The listing builds one solid part. Answer for the finished solid, in the listing's coordinates (mm). A direction names the side the tool comes from. Coordinates: 2 decimals unless noted, no trailing zeros. Loops run counter-clockwise (first coordinate to the right, second up) from the corner with the lowest first, then second, coordinate; pieces in that order, holes last. Notation, with made-up numbers: M -10,77 L 13,77 A34 cw 13,116 Z; hole C 57.5,11 d2. An arc over 180 degrees is marked long. Return JSON: item names as keys, results as strings. Group by question number.
1. Section A-A (x = -78) is taken. Write down the section's boundary in (y, z).
2. Section B-B (y = -24.5) is taken. Write down the section's boundary in (x, z), then the cut area to 3 significant figures.
3. Section D-D (y = 97.5) is taken. Write down the section's boundary in (x, z), then the cut area to 3 significant figures.
4. Which of the six approach directions +Z, -Z, +X, -X, +Y, -Y give full straight-line access (tool end or side, diameter ignored) to faces 5 (the face through (54.8, 38, 0.5)), 6 (the face through (-46, 32, 1))?
5. Straight lines are drawn through the part: L1, parallel to X at y = -25, z = 0.9; L2, parallel to X at y = -42.5, z = 0.3; L3, parallel to Y at x = -80.5, z = 0.65. For each, find the intervals that lie inside material, in ascending order. Write a range as from..to.
6. The mould has two halves that part along X. Classify faces 1 (the face through (-91, -49, 0.5)), 2 (the face through (104.27, -47.94, 0.49)), 3 (the face through (-46, 32, 0)), 4 (the face through (6.155, -50.41, 0.493)): pulls with the +X half, pulls with the -X half, needs draft (parallel to the pull), parting line crosses it, or undercut.
7. Section C-C (x = -172) is taken. Write down the section's boundary in (y, z).
```python
from build123d import *

# Parameters (mm, degrees)
ESQUISSE2_R             = 21.716757685
BOSS_EXTRU_1_DEPTH      = 1
ENL_V_MAT_EXTRU_2_DEPTH = 293.837814183
CONG_2_R                = 10
CONG_3_R                = 6
CONG_4_R                = 6
CONG_5_R                = 6


with BuildPart() as part:
    # Esquisse2 → Boss.-Extru.1 (new body)
    with BuildSketch(Plane.XY):
        with Locations((-43.22899501, 36.585487108)):
            Circle(ESQUISSE2_R)
        with BuildLine():
            ThreePointArc((-207.546192285, -7.001881243), (-132.259115873, 40.696309579), (-43.22899501, 36.585487108))
            ThreePointArc((-43.22899501, 36.585487108), (-84.183978752, -42.572270496), (-163.135361924, -83.923695834))
            ThreePointArc((-163.135361924, -83.923695834), (-190.453313653, -48.414512892), (-207.546192285, -7.001881243))
        make_face()
        with BuildLine():
            ThreePointArc((76.677371904, -83.923695834), (-2.274011269, -42.572270496), (-43.22899501, 36.585487108))
            ThreePointArc((-43.22899501, 36.585487108), (45.801125853, 40.696309579), (121.088202265, -7.001881243))
            ThreePointArc((121.088202265, -7.001881243), (103.995323633, -48.414512892), (76.677371904, -83.923695834))
        make_face()
        with BuildLine():
            Line((-43.22899501, 206.585487108), (-43.22899501, 58.302244794))
            ThreePointArc((-43.22899501, 58.302244794), (-34.753748483, 56.580180421), (-27.622617897, 51.687094896))
            ThreePointArc((-27.622617897, 51.687094896), (7.298277527, 122.217794206), (1.181835351, 200.682038403))
            ThreePointArc((1.181835351, 200.682038403), (-20.82825529, 205.103162324), (-43.22899501, 206.585487108))
        make_face()
        with BuildLine():
            ThreePointArc((-58.835372123, 51.687094896), (-51.704241537, 56.580180421), (-43.22899501, 58.302244794))
            Line((-43.22899501, 58.302244794), (-43.22899501, 206.585487108))
            ThreePointArc((-43.22899501, 206.585487108), (-65.62973473, 205.103162324), (-87.639825371, 200.682038403))
            ThreePointArc((-87.639825371, 200.682038403), (-93.756267547, 122.217794206), (-58.835372123, 51.687094896))
        make_face()
        with BuildLine():
            ThreePointArc((-48.504182436, 15.519164174), (-45.480177087, 25.955564863), (-43.22899501, 36.585487108))
            ThreePointArc((-43.22899501, 36.585487108), (-53.560368754, 39.950867364), (-64.110559549, 42.550202255))
            ThreePointArc((-64.110559549, 42.550202255), (-62.036258854, 25.727108266), (-48.504182436, 15.519164174))
        make_face()
        with BuildLine():
            ThreePointArc((-22.347430471, 42.550202255), (-32.897621267, 39.950867364), (-43.22899501, 36.585487108))
            ThreePointArc((-43.22899501, 36.585487108), (-40.977812933, 25.955564863), (-37.953807584, 15.519164174))
            ThreePointArc((-37.953807584, 15.519164174), (-26.109159563, 23.224020174), (-21.512237325, 36.585487108))
            ThreePointArc((-21.512237325, 36.585487108), (-21.722049137, 39.596939182), (-22.347430471, 42.550202255))
        make_face()
        with BuildLine():
            ThreePointArc((-37.953807584, 15.519164174), (-40.977812933, 25.955564863), (-43.22899501, 36.585487108))
            ThreePointArc((-43.22899501, 36.585487108), (-45.480177087, 25.955564863), (-48.504182436, 15.519164174))
            ThreePointArc((-48.504182436, 15.519164174), (-43.22899501, 14.868729423), (-37.953807584, 15.519164174))
        make_face()
        with BuildLine():
            ThreePointArc((-64.110559549, 42.550202255), (-53.560368754, 39.950867364), (-43.22899501, 36.585487108))
            ThreePointArc((-43.22899501, 36.585487108), (-51.309186676, 43.850029099), (-58.835372123, 51.687094896))
            ThreePointArc((-58.835372123, 51.687094896), (-62.036258854, 47.443865951), (-64.110559549, 42.550202255))
        make_face()
        with BuildLine():
            ThreePointArc((-58.835372123, 51.687094896), (-51.309186676, 43.850029099), (-43.22899501, 36.585487108))
            Line((-43.22899501, 36.585487108), (-43.22899501, 58.302244794))
            ThreePointArc((-43.22899501, 58.302244794), (-51.704241537, 56.580180421), (-58.835372123, 51.687094896))
        make_face()
        with BuildLine():
            Line((-43.22899501, 58.302244794), (-43.22899501, 36.585487108))
            ThreePointArc((-43.22899501, 36.585487108), (-35.148803344, 43.850029099), (-27.622617897, 51.687094896))
            ThreePointArc((-27.622617897, 51.687094896), (-34.753748483, 56.580180421), (-43.22899501, 58.302244794))
        make_face()
        with BuildLine():
            ThreePointArc((-27.622617897, 51.687094896), (-35.148803344, 43.850029099), (-43.22899501, 36.585487108))
            ThreePointArc((-43.22899501, 36.585487108), (-32.897621267, 39.950867364), (-22.347430471, 42.550202255))
            ThreePointArc((-22.347430471, 42.550202255), (-24.421731167, 47.443865951), (-27.622617897, 51.687094896))
        make_face()
    extrude(amount=BOSS_EXTRU_1_DEPTH)

    # Esquisse4 → Enlèv. mat.-Extru.2 (cut, through all)
    with BuildSketch(Plane(origin=(0, 0, 0), x_dir=(-1, 0, 0), z_dir=(0, 0, -1))):
        with BuildLine():
            Line((46.937094254, 35.085487108), (39.520895767, 35.085487108))
            ThreePointArc((39.520895767, 35.085487108), (43.22899501, 40.585487108), (46.937094254, 35.085487108))
        make_face()
    extrude(amount=-ENL_V_MAT_EXTRU_2_DEPTH, mode=Mode.SUBTRACT)

    # Congé2
    cong_2_edges = [part.edges().sort_by_distance(p)[0] for p in [
        (-87.639825371, 200.682038403, 0.5),
        (1.181835351, 200.682038403, 0.5),
        (121.088202265, -7.001881243, 0.5),
        (76.677371904, -83.923695834, 0.5),
        (-163.135361924, -83.923695834, 0.5),
        (-207.546192285, -7.001881243, 0.5),
    ]]
    fillet(cong_2_edges, radius=CONG_2_R)

    # Congé3
    cong_3_edges = [part.edges().sort_by_distance(p)[0] for p in [
        (-64.110559549, 42.550202255, 0.5),
        (-58.835372123, 51.687094896, 0.5),
    ]]
    fillet(cong_3_edges, radius=CONG_3_R)

    # Congé4
    cong_4_edges = [part.edges().sort_by_distance(p)[0] for p in [
        (-27.622617897, 51.687094896, 0.5),
        (-22.347430471, 42.550202255, 0.5),
    ]]
    fillet(cong_4_edges, radius=CONG_4_R)

    # Congé5
    cong_5_edges = [part.edges().sort_by_distance(p)[0] for p in [
        (-37.953807584, 15.519164174, 0.5),
        (-48.504182436, 15.519164174, 0.5),
    ]]
    fillet(cong_5_edges, radius=CONG_5_R)


solid = part.part
```
Worked out:
{
 "1": {"outline": "M -35.97,0 L 44.76,0 L 44.76,1 L -35.97,1 Z; M 78.74,0 L 202.99,0 L 202.99,1 L 78.74,1 Z"},
 "2": {"outline": "M -201.88,0 L -68.87,0 L -68.87,1 L -201.88,1 Z; M -17.59,0 L 115.42,0 L 115.42,1 L -17.59,1 Z", "area": "266 mm^2"},
 "3": {"outline": "M -86.71,0 L 0.25,0 L 0.25,1 L -86.71,1 Z", "area": "87.0 mm^2"},
 "4": {"face 5": "+Z, -Z", "face 6": "+Z, +X, -X, +Y, -Y"},
 "5": {"L1": "-201.68..-69.23, -17.22..115.22", "L2": "-193.71..-84.11, -2.35..107.26", "L3": "-38.73..45.01, 83.47..202.45"},
 "6": {"face 1": "undercut", "face 2": "pulls with the +X half", "face 3": "needs draft", "face 4": "undercut"},
 "7": {"outline": "M -74.4,0 L 23.62,0 L 23.62,1 L -74.4,1 Z"}
}
